The listing builds one solid part. Answer for the finished solid, in the listing's coordinates (mm). Coordinates: 2 decimals unless noted, no trailing zeros. Order: outer loops, then holes, each group sorted by start corner. A loop starts at its lowest first (then second) coordinate and runs counter-clockwise, first axis right, second up. Notation, with made-up numbers: (75.5, 0.5) -> (117.5, 0.5) arc R18 ccw to (117.5, 27.5) -> close; hole circle Ø2 at (74, 0). An arc over 180 degrees is marked (long way). Return JSON: item names as keys, results as strings.
Autodesk Inventor part; units mm, degrees
ref_plane "YZ Plane" through (0, 0, 0) normal (1, 0, 0) x (0, 1, 0)
ref_plane "XZ Plane" through (0, 0, 0) normal (0, 1, 0) x (-1, 0, 0)
ref_plane "XY Plane" through (0, 0, 0) normal (0, 0, 1) x (1, 0, 0)
sketch "スケッチ1" plane through (0, 0, 0) normal (0, 0, 1) x (1, 0, 0)
  circle A0 centre (0, 0) radius 23.45
  circle A1 centre (0, 0) radius 36.55
  line L0 (0, 0) -> (-28.1908, 10.2606) construction
  line L1 (0, 0) -> (28.1908, 10.2606) construction
  line L2 (-39.5959, 0) -> (43.1917, 0) construction
  line L3 (0, 0) -> (0, 30) construction
  circle A2 centre (-28.1908, 10.2606) radius 2.55
  circle A3 centre (0, 30) radius 2.55
  circle A4 centre (28.1908, 10.2606) radius 2.55
  dimension "d0" = 73.1
  dimension "d1" = 46.9
  dimension "d2" = 30
  dimension "d3" = 30
  dimension "d6" = 20
  dimension "d7" = 20
  dimension "d8" = 30
  dimension "d9" = 5.1
  dimension "d10" = 5.1
  dimension "d11" = 5.1
extrude "押し出し1" add sketch "スケッチ1" along normal blind 10
sketch "スケッチ2" plane through (0, 0, 10) normal (0, 0, 1) x (1, 0, 0)
  line L0 (0, 0) -> (0, -80) construction
  circle A0 centre (0, -80) radius 52.5
  dimension "d14" = 80
  dimension "d18" = 105
extrude "押し出し2" cut sketch "スケッチ2" against normal blind 10
sketch "スケッチ3" plane through (0, 0, 10) normal (0, 0, 1) x (1, 0, 0)
  circle A0 centre (28.1908, 10.2606) radius 2.55
  line L0 (0, 0) -> (28.1908, 10.2606)
  circle A1 centre (-28.1908, 10.2606) radius 2.55
  line L1 (-28.1908, 10.2606) -> (0, 0)
  circle A2 centre (0, 30) radius 2.55
  line L2 (0, 0) -> (0, 30)
properties part number "円 46.9mm"
1. Each of these flat-tipped pins is pushed along its axis until it touches: pin 1 Ø3 at (x, y) = (-28.19, 10.26) entering from +Z; pin 2 Ø1 at (x, z) = (-12, 7) entering from -Y; pin 3 Ø1.5 at (y, z) = (10.5, 7.5) entering from -X; pin 4 Ø1 at (y, z) = (-13, 4.5) entering from -X. Where does it stop, or does it pass through?
Answer block:
{"pin 1": "passes through", "pin 2": "stops at y = -29.01", "pin 3": "stops at x = -35.23", "pin 4": "stops at x = -34.35"}
2. The part is cut by section B-B on y = 0. Give the vertices of the cut face in (x, z).
Answer block:
{"outline": "(-36.55, 0) -> (-23.45, 0) -> (-23.45, 10) -> (-36.55, 10) -> close; (23.45, 0) -> (36.55, 0) -> (36.55, 10) -> (23.45, 10) -> close"}
3. Consider line 1 (Y direction, x = 0, z = 7.75); line 2 (X direction, y = 12.5, z = 6.25); line 3 (X direction, y = 10, z = 5). Determine where each line is inside the solid, lowest interval first. Write a range as from..to.
Answer block:
{"line 1": "y = -27.5..-23.45, 23.45..27.45, 32.55..36.55", "line 2": "x = -34.35..-29.41, -26.97..-19.84, 19.84..26.97, 29.41..34.35", "line 3": "x = -35.16..-30.73, -25.65..-21.21, 21.21..25.65, 30.73..35.16"}
4. The part is cut by section A-A on x = 0. Give the vertices of the cut face in (y, z).
Answer block:
{"outline": "(-27.5, 0) -> (-23.45, 0) -> (-23.45, 10) -> (-27.5, 10) -> close; (23.45, 0) -> (27.45, 0) -> (27.45, 10) -> (23.45, 10) -> close; (32.55, 0) -> (36.55, 0) -> (36.55, 10) -> (32.55, 10) -> close"}
5. The part is cut by section D-D on z = 5. Give the vertices of the cut face in (x, y), and give its area (3 significant figures).
Answer block:
{"outline": "(-19.16, -31.12) arc R52.5 cw to (19.16, -31.12) arc R36.55 ccw (long way) to start; hole circle Ø5.1 at (-28.19, 10.26); hole circle Ø46.9 at (0, 0); hole circle Ø5.1 at (0, 30); hole circle Ø5.1 at (28.19, 10.26)", "area": "2,170 mm2"}
6. The part is cut by section C-C on x = 15. Give the vertices of the cut face in (y, z), and give its area (3 significant figures).
Answer block:
{"outline": "(-29.69, 0) -> (-18.03, 0) -> (-18.03, 10) -> (-29.69, 10) -> close; (18.03, 0) -> (33.33, 0) -> (33.33, 10) -> (18.03, 10) -> close", "area": "270 mm2"}
7. Determine the mould class of faces 1 (the face through (16, 18, 10)), 2 (the face through (-1.325, 36.526, 4.93)), 3 (the face through (-25.76, 9.49, 4.93)) for opening direction X: pulls with the +X half, pulls with the -X half, needs draft (parallel to the pull), parting line crosses it, or undercut.
Answer block:
{"face 1": "needs draft", "face 2": "parting line crosses it", "face 3": "undercut"}
